Verification items for the finished model (mm, model axes). Round coordinates to 2 decimals unless told otherwise and drop trailing zeros. Loops run counter-clockwise (first coordinate to the right, second up) from the corner with the lowest first, then second, coordinate; pieces in that order, holes last. Notation, with made-up numbers: M 58.5,6.25 L 73.5,6.25 A23 cw 73.5,20.25 Z; hole C -17,78.25 d6. An arc over 180 degrees is marked long. One line per item, written item: value.
from build123d import *

# Parameters (mm, degrees)
SKETCH3_R           = 1.5
BOSS_EXTRUDE1_DEPTH = 9
SKETCH4_R           = 3.5
BOSS_EXTRUDE2_DEPTH = 1.75
FILLET3_R           = 0.75
CUT_EXTRUDE4_DEPTH  = 0.75
FILLET4_R           = 0.25


with BuildPart() as part:
    # Sketch3 → Boss-Extrude1 (new body)
    with BuildSketch(Plane(origin=(0, 0, 0), x_dir=(1, 0, 0), z_dir=(0, 1, 0))):
        with Locations(Location((0, 0, 0), (0, 0, 270))):
            Circle(SKETCH3_R)
    extrude(amount=BOSS_EXTRUDE1_DEPTH)

    # Sketch4 → Boss-Extrude2 (add)
    with BuildSketch(Plane(origin=(0, 9, 0), x_dir=(1, 0, 0), z_dir=(0, 1, 0))):
        with Locations(Location((0, 0, 0), (0, 0, 270))):
            Circle(SKETCH4_R)
    extrude(amount=BOSS_EXTRUDE2_DEPTH)

    # Fillet3
    fillet3_edges = [part.edges().sort_by_distance(p)[0] for p in [
        (0, 10.75, -3.5),
    ]]
    fillet(fillet3_edges, radius=FILLET3_R)

    # Sketch6 → Cut-Extrude4 (cut)
    with BuildSketch(Plane(origin=(0, 10.75, 0), x_dir=(1, 0, 0), z_dir=(0, 1, 0))):
        Polygon((0.425, 0.425), (2, 0.425), (2, -0.425), (0.425, -0.425), (0.425, -2), (-0.425, -2), (-0.425, -0.425), (-2, -0.425), (-2, 0.425), (-0.425, 0.425), (-0.425, 2), (0.425, 2), align=None)
    extrude(amount=-CUT_EXTRUDE4_DEPTH, mode=Mode.SUBTRACT)

    # Fillet4
    fillet4_edges = [part.edges().sort_by_distance(p)[0] for p in [
        (0, 9, -1.5),
    ]]
    fillet(fillet4_edges, radius=FILLET4_R)


solid = part.part
(1) Depth check by flat-ended pin: pin 1 Ø0.8 at (y, z) = (10.5, -1.5) entering from +X; pin 2 Ø3 at (x, z) = (1, 0) entering from +Y; pin 3 Ø0.6 at (y, z) = (10.5, 0) entering from +X; pin 4 Ø0.6 at (x, y) = (0, 10.5) entering from -Z. Enter the tip coordinate at first touch or a pass-through.
Completed:
pin 1: stops at x = 3.25
pin 2: stops at y = 10.75
pin 3: stops at x = 3.47
pin 4: stops at z = -3.47
(2) Sectioned sample at B-B on z = 0. Enter the section's corners in (x, y), and give its area (3 significant figures).
Completed:
outline: M -3.5,9 L -1.75,9 A0.25 cw -1.5,8.75 L -1.5,0 L 1.5,0 L 1.5,8.75 A0.25 cw 1.75,9 L 3.5,9 L 3.5,10 A0.75 ccw 2.75,10.75 L 2,10.75 L 2,10 L -2,10 L -2,10.75 L -2.75,10.75 A0.75 ccw -3.5,10 Z
area: 36.0 mm^2
(3) Sectioned sample at C-C on y = 4.5. Enter the section's corners in (x, z).
Completed:
outline: C 0,0 d3
(4) Thickness scan on L1, parallel to Y at x = -2, z = 1.75; L2, parallel to Z at x = -0.5, y = 10.25 (3 decimals); L3, parallel to Y at x = 0, z = 0. Record the ranges inside material, lowest first. Write a range as from..to.
Completed:
L1: y = 9..10.75
L2: z = -3.421..-0.425, 0.425..3.421
L3: y = 0..10
(5) Mould release check, pull along Y, two halves, no side actions. Record for faces 1 (the face through (-1, 10.75, 1)), 2 (the face through (2, 9, 1)), 3 (the face through (0.45, 4.31, 1.43)): +Y half, -Y half, draft (parallel to the pull), parting line (faces both ways), or undercut.
Completed:
face 1: +Y half
face 2: -Y half
face 3: draft
(6) Sectioned sample at A-A on x = 0. Enter the section's corners in (y, z), and give its area (3 significant figures).
Completed:
outline: M 0,-1.5 L 8.75,-1.5 A0.25 cw 9,-1.75 L 9,-3.5 L 10,-3.5 A0.75 ccw 10.75,-2.75 L 10.75,-2 L 10,-2 L 10,2 L 10.75,2 L 10.75,2.75 A0.75 ccw 10,3.5 L 9,3.5 L 9,1.75 A0.25 cw 8.75,1.5 L 0,1.5 Z
area: 36.0 mm^2
